The model under review builds one solid part; all positions refer to its coordinate system, in mm. A direction names the side the tool comes from. Round coordinates to 2 decimals unless told otherwise and drop trailing zeros. Order: outer loops, then holes, each group sorted by start corner. A loop starts at its lowest first (then second) coordinate and runs counter-clockwise, first axis right, second up.
```python
from build123d import *

# Parameters (mm, degrees)
PAD_DEPTH       = 35
POCKET_DEPTH    = 8
POCKET001_DEPTH = 8
SKETCH003_R     = 2.207749
POCKET002_DEPTH = 8.001
SKETCH004_W     = 29.275187
SKETCH004_H     = 26.084862
POCKET003_DEPTH = 29


with BuildPart() as part:
    # Sketch → Pad (new body, symmetric)
    with BuildSketch(Plane.XY):
        Polygon((-37.608468, 25.834033), (-37.608468, -30.264225), (82.694635, -30.264225), align=None)
    extrude(amount=PAD_DEPTH, both=True)

    # Sketch001 → Pocket (cut)
    with BuildSketch(Plane.XY.offset(35)):
        Polygon((-37.608468, 25.834033), (-37.608468, -22.264225), (65.538579, -22.264225), align=None)
    extrude(amount=-POCKET_DEPTH, mode=Mode.SUBTRACT)

    # Sketch002 → Pocket001 (cut)
    with BuildSketch(Plane(origin=(0, 0, -35), x_dir=(1, 0, 0), z_dir=(0, 0, -1))):
        Polygon((65.538579, 22.264225), (-37.608468, 22.264225), (-37.608468, -25.834033), align=None)
    extrude(amount=-POCKET001_DEPTH, mode=Mode.SUBTRACT)

    # Sketch003 → Pocket002 (cut, through all)
    with BuildSketch(Plane(origin=(0, -22.264225, 0), x_dir=(-1, 0, 0), z_dir=(0, 1, 0))):
        with Locations((-52.391532, 31)):
            Circle(SKETCH003_R)
        with Locations((27.608468, 31)):
            Circle(SKETCH003_R)
        with Locations((-52.391532, -31)):
            Circle(SKETCH003_R)
        with Locations((27.608468, -31)):
            Circle(SKETCH003_R)
    extrude(amount=-POCKET002_DEPTH, mode=Mode.SUBTRACT)

    # Sketch004 → Pocket003 (cut)
    with BuildSketch(Plane.XZ.offset(30.264225)):
        with Locations((-14.936289, 0)):
            Rectangle(SKETCH004_W, SKETCH004_H)
    extrude(amount=-POCKET003_DEPTH, mode=Mode.SUBTRACT)


solid = part.part
```
(1) To check wall thickness, follow probe 1 along Z at (x, y) = (-8, -26); probe 2 along Z at (x, y) = (-20.5, 17); probe 3 along X at (y, z) = (-27, 10). State the ranges of each line that lie inside material, in increasing order.
Data:
probe 1: z = -35 to -13.04, 13.04 to 35
probe 2: z = -27 to 27
probe 3: x = -37.61 to -29.57, -0.3 to 75.69
(2) Consider section A-A (z = 31). Write out the cut boundary in (x, y), and give its area (3 significant figures).
Data:
outline: (-37.61, -30.26) - (-29.82, -30.26) - (-29.82, -22.26) - (-37.61, -22.26) - close; (-25.4, -30.26) - (50.18, -30.26) - (50.18, -22.26) - (-25.4, -22.26) - close; (54.6, -30.26) - (82.69, -30.26) - (65.54, -22.26) - (54.6, -22.26) - close
area: 823 mm2
(3) Consider section B-B (x = 1.5). Write out the cut boundary in (y, z), and give its area (3 significant figures).
Data:
outline: (-30.26, -35) - (-22.26, -35) - (-22.26, -27) - (7.6, -27) - (7.6, 27) - (-22.26, 27) - (-22.26, 35) - (-30.26, 35) - close
area: 2,170 mm2
(4) Draft analysis for pull direction X (two halves, no side actions). For faces 1 (the flat face through (22, -30.264, 0)), 2 (the flat face through (-37.608, -2, 0)), 3 (the flat face through (-29.574, -16, 0)), state which applies: pulls with the +X half, pulls with the -X half, needs draft (parallel to the pull), parting line crosses it, or undercut.
Data:
face 1: needs draft
face 2: pulls with the -X half
face 3: undercut
(5) Insertion check: pin 1 (8 mm diameter, centred on x = -3.5, y = 15.5, fed in from -Z); pin 2 (14.5 mm diameter, centred on x = -3, y = -9.5, fed in from +Z); pin 3 (8 mm diameter, centred on x = 10.5, y = -16, fed in from -Z); pin 4 (12 mm diameter, centred on y = 14, z = -15.5, fed in from +X). Each pin has a flat end and moves straight along its axis. Give the tip position at first contact, or say it passes through.
Data:
pin 1: passes through
pin 2: stops at z = 27
pin 3: stops at z = -27
pin 4: stops at x = 0.64
(6) For faces 4 (the flat face through (15, -22.264, -31)), 5 (the flat face through (13, -22.264, 31)), 6 (the flat face through (-15, -16, -13.042)), list the 3-axis set-ups (+Z, -Z, +X, -X, +Y, -Y) from which the entire face can be reached by the end or side of a thin tool; tool diameter is ignored.
Data:
face 4: -Z, +X, -X, +Y
face 5: +Z, +X, -X, +Y
face 6: -Y
(7) Consider section C-C (z = 2). Write out the cut boundary in (x, y).
Data:
outline: (-37.61, -30.26) - (-29.57, -30.26) - (-29.57, -1.26) - (-0.3, -1.26) - (-0.3, -30.26) - (82.69, -30.26) - (-37.61, 25.83) - close
(8) Consider section D-D (y = -17.5). Write out the cut boundary in (x, z).
Data:
outline: (-37.61, -27) - (55.32, -27) - (55.32, 27) - (-37.61, 27) - close; hole (-29.57, -13.04) - (-0.3, -13.04) - (-0.3, 13.04) - (-29.57, 13.04) - close
